Source: CAD feature listing. Evaluate the final solid. Frame: model axes, mm. A direction names the side the tool comes from. Give positions to 0.01 mm unless a question says otherwise; leave off trailing zeros. Loops run counter-clockwise (first coordinate to the right, second up) from the corner with the lowest first, then second, coordinate; pieces in that order, holes last. Notation, with made-up numbers: M 18,82.5 L 42,82.5 A27 ccw 42,115.5 Z; hole C -30.75,18.25 d4. An arc over 180 degrees is marked long. Answer in a Markdown table with one row per item.
```python
from build123d import *

# Parameters (mm, degrees)
BOSS_EXTRUDE1_DEPTH = 3
TAPPED_HOLE1_D      = 3.3
CHAMFER1_SIZE       = 0.4
SKETCH5_W           = 0.75
SKETCH5_H           = 0.8
FILLET1_R           = 0.2


with BuildPart() as part:
    # Sketch1 → Boss-Extrude1 (new body)
    with BuildSketch(Plane(origin=(0, 0, 0), x_dir=(1, 0, 0), z_dir=(0, 1, 0))):
        Polygon((0, 4.041451884), (-3.5, 2.020725942), (-3.5, -2.020725942), (0, -4.041451884), (3.5, -2.020725942), (3.5, 2.020725942), align=None)
    extrude(amount=-BOSS_EXTRUDE1_DEPTH)

    # Sketch2 → Cut-Revolve1 (revolve, cut)
    with BuildSketch(Plane(origin=(0, 0, 0), x_dir=(0, 0, -1), z_dir=(1, 0, 0))):
        Polygon((3.5, 0), (4.041451884, 0), (4.041451884, -0.145081595), align=None)
        Polygon((4.041451884, -2.854918405), (3.5, -3), (4.041451884, -3), align=None)
    revolve(axis=Axis((0, 0, 0), (0, -1, 0)), mode=Mode.SUBTRACT)

    # Tapped Hole1 (through all)
    with Locations(Plane(origin=(0, 0, 0), x_dir=(1, 0, 0), z_dir=(0, 1, 0))):
        with Locations((0, 0)):
            Hole(TAPPED_HOLE1_D / 2)

    # Chamfer1
    chamfer1_edges = [part.edges().sort_by_distance(p)[0] for p in [
        (1.65, 0, 0),
        (1.65, -3, 0),
    ]]
    chamfer(chamfer1_edges, length=CHAMFER1_SIZE)

    # Sketch5 → Revolve1 (revolve)
    with BuildSketch(Plane.XY, mode=Mode.PRIVATE) as revolve1_sk:
        with Locations((3.125, 0.4)):
            Rectangle(SKETCH5_W, SKETCH5_H)
    revolve(revolve1_sk.sketch.rotate(Axis((0, 0, 0), (0, 1, 0)), 270), axis=Axis((0, 0, 0), (0, 1, 0)))

    # Fillet1
    fillet1_edges = [part.edges().sort_by_distance(p)[0] for p in [
        (0, 0.8, -3.5),
    ]]
    fillet(fillet1_edges, radius=FILLET1_R)


solid = part.part
```
Q1. Contact query for a flat-ended pin moving along its axis: pin 1 Ø3.5 at (x, z) = (0, 0) entering from -Y. Output: stop coordinate, or through.
Values follow:
| item | result |
|---|---|
| pin 1 | y = -2.7 |
Q2. Section query A-A (y = -1.7). Output: boundary loops of the cut face in (x, z).
Values follow:
| item | result |
|---|---|
| outline | M -3.5,-2.02 L 0,-4.04 L 3.5,-2.02 L 3.5,2.02 L 0,4.04 L -3.5,2.02 Z; hole C 0,0 d3.3 |
Q3. Mould query, pull axis X, two halves, no side actions, for faces 1 (the flat face through (-1.8, -1.5, 3)), 2 (the cylindrical face through (2.95, 0.3, 1.88)), 3 (the flat face through (-1, 0, 2)), 4 (the conical face through (3.19, -0.05, -1.85)). Classes: +X half, -X half, draft (parallel to the pull), parting line (faces both ways), or undercut.
Values follow:
| item | result |
|---|---|
| face 1 | -X half |
| face 2 | parting line |
| face 3 | undercut |
| face 4 | +X half |
Q4. Reachability of faces 5 (the conical face through (3.19, -2.95, -1.85)), 6 (the cylindrical face through (-2.685, 0.406, -0.596)) from +Z, -Z, +X, -X, +Y, -Y: full face, straight path, thin tool, end or side. Return the list, or none.
Values follow:
| item | result |
|---|---|
| face 5 | -Z, +X, -Y |
| face 6 | +Y |
Q5. Section query B-B (y = -0.3). Output: boundary loops of the cut face in (x, z), plus the area to 3 significant figures.
Values follow:
| item | result |
|---|---|
| outline | M -3.5,-2.02 L 0,-4.04 L 3.5,-2.02 L 3.5,2.02 L 0,4.04 L -3.5,2.02 Z; hole C 0,0 d3.5 |
| area | 32.8 mm^2 |
Q6. Ray query, probe 1 along X at (y, z) = (0.4, 0); probe 2 along Y at (x, z) = (-2.5, -0.5); probe 3 along Z at (x, y) = (-2.5, 0.35). Return the intervals inside material, ascending. Write a range as from..to.
Values follow:
| item | result |
|---|---|
| probe 1 | -3.5..-2.75, 2.75..3.5 |
| probe 2 | -3..0 |
| probe 3 | -2.45..-1.15, 1.15..2.45 |
